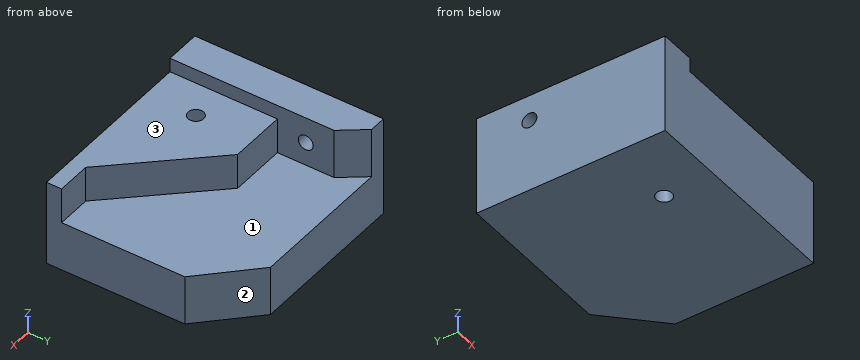
Autodesk Fusion 360 part; units mm, degrees
sketch "Sketch1" plane through (0, 0, 0) normal (0, 0, 1) x (1, 0, 0)
  line L0 (0, 0) -> (174.2555, 0)
  line L1 (174.2555, 0) -> (174.2555, 132.964)
  line L2 (174.2555, 132.964) -> (0, 132.964)
  line L3 (0, 132.964) -> (0, 0)
  line L4 (138.7597, 132.964) -> (174.2555, 97.4682)
  line L5 (138.7597, 132.964) -> (188.9583, 132.964) construction
  dimension "d1" = 45
extrude "Extrude1" add sketch "Sketch1" along normal blind 35 contours L0 L1 L2 L3 L4
extrude "Extrude2" cut 1 faces at (0, 88.6427, 11.6667) along direction (1, 0, 0) blind 25
sketch "Sketch2" plane through (0, 0, 35) normal (0, 0, 1) x (-1, 0, 0)
  line L0 (-25, -132.964) -> (-25, 0)
  line L1 (-25, 0) -> (-174.2555, 0)
  line L2 (-174.2555, 0) -> (-174.2555, -97.4682)
  line L3 (-174.2555, -97.4682) -> (-138.7597, -132.964)
  line L4 (-138.7597, -132.964) -> (-25, -132.964)
  line L5 (-25, -132.964) -> (-25, 0)
  line L6 (-50, 0) -> (-50, -110)
  line L7 (-50, -110) -> (-50, -115.7208)
  line L8 (-50, -115.7208) -> (-36.875, -132.964)
extrude "Extrude3" add sketch "Sketch2" along normal blind 35 contours L0 L1 L4 L5 L6 L7 L8
sketch "Sketch3" plane through (0, 0, 35) normal (0, 0, 1) x (-1, 0, 0)
  line L0 (-36.875, -132.964) -> (-50, -115.7208)
  line L1 (-50, -115.7208) -> (-50, 0)
  line L2 (-50, 0) -> (-174.2555, 0)
  line L3 (-174.2555, 0) -> (-174.2555, -97.4682)
  line L4 (-174.2555, -97.4682) -> (-138.7597, -132.964)
  line L5 (-138.7597, -132.964) -> (-36.875, -132.964)
  line L6 (-174.2555, -10.6135) -> (-155, -10.6135)
  line L7 (-50, 0) -> (-174.2555, 0)
  line L8 (-155, -10.6135) -> (-150, -10.6135)
  line L9 (-50, -75.7001) -> (-90, -75.7001)
  line L10 (-90, -75.7001) -> (-150, -10.6135)
extrude "Extrude4" add sketch "Sketch3" along normal blind 25 contours L1 L2 L3 L6 L7 L8 L9 L10
sketch "Sketch4" plane through (50, 0, 0) normal (1, 0, 0) x (0, 1, 0)
  line L0 (75.7001, 60) -> (75.7001, 35)
  line L1 (75.7001, 35) -> (115.7208, 35)
  line L2 (115.7208, 35) -> (115.7208, 70)
  line L3 (115.7208, 70) -> (0, 70)
  line L4 (0, 70) -> (0, 60)
  line L5 (0, 60) -> (75.7001, 60)
  circle A0 centre (95.7105, 51.6698) radius 5.2582
extrude "Extrude5" cut sketch "Sketch4" against normal blind 50 contours A0
sketch "Sketch5" plane through (0, 0, 60) normal (0, 0, 1) x (-1, 0, 0)
  line L0 (-174.2555, -10.6135) -> (-150, -10.6135)
  line L1 (-150, -10.6135) -> (-90, -75.7001)
  line L2 (-90, -75.7001) -> (-50, -75.7001)
  line L3 (-50, -75.7001) -> (-50, 0)
  line L4 (-50, 0) -> (-174.2555, 0)
  line L5 (-174.2555, 0) -> (-174.2555, -10.6135)
  circle A0 centre (-74.3342, -35.2984) radius 5.4818
extrude "Extrude6" cut sketch "Sketch5" against normal blind 150 contours A0
Verification items for the finished model (mm, model axes). Face numbers are marked on the shaded views. A direction names the side the tool comes from. Give positions to 0.01 mm unless a question says otherwise; leave off trailing zeros. Loops run counter-clockwise (first coordinate to the right, second up) from the corner with the lowest first, then second, coordinate; pieces in that order, holes last.
1. Section check A-A, the plane z = 53.5. Enter the section's corners in (x, y) (1 decimal).
2. Set-up check for the marked faces 1, 2 and 3: record each of +Z, -Z, +X, -X, +Y, -Y from which the full face is reachable in a straight line by a thin tool's end or side.
3. Section check C-C, the plane x = 72. Enter the section's corners in (y, z).
4. Section check D-D, the plane z = 38.5. Enter the section's corners in (x, y) (1 decimal), then the cut area to 3 significant figures.
5. Section check B-B, the plane y = 93.5. Enter the section's corners in (x, z).
6. Thickness scan on line 1 (Z direction, x = 123, y = 91); line 2 (Z direction, x = 99.5, y = 33); line 3 (X direction, y = 98.5, z = 64.5). Record the ranges inside material, lowest first.
7. Go/stop test with flat-tipped pins: pin 1 Ø10.5 at (y, z) = (65.5, 50) entering from +X; pin 2 Ø22.5 at (x, y) = (119.5, 43) entering from +Z; pin 3 Ø19.5 at (x, z) = (165, 45.5) entering from +Y; pin 4 Ø8 at (x, z) = (68, 19) entering from -Y. Record where each tip stops, or that it passes through.
Geometry says:
1. outline: (25, 0) - (174.3, 0) - (174.3, 10.6) - (150, 10.6) - (90, 75.7) - (50, 75.7) - (50, 90.8) - (25, 90.8) - close; (25, 100.6) - (50, 100.6) - (50, 115.7) - (36.9, 133) - (25, 133) - close; hole circle Ø11 at (74.3, 35.3)
2. face 1: +Z, +X, +Y
2. face 2: +Z, -Z, +X, +Y
2. face 3: +Z, +X, +Y, -Y
3. outline: (0, 0) - (30.34, 0) - (30.34, 60) - (0, 60) - close; (40.26, 0) - (132.96, 0) - (132.96, 35) - (75.7, 35) - (75.7, 60) - (40.26, 60) - close
4. outline: (25, 0) - (174.3, 0) - (174.3, 10.6) - (150, 10.6) - (90, 75.7) - (50, 75.7) - (50, 115.7) - (36.9, 133) - (25, 133) - close; hole circle Ø11 at (74.3, 35.3)
4. area: 8,990 mm2
5. outline: (25, 0) - (174.26, 0) - (174.26, 35) - (50, 35) - (50, 46.9) - (25, 46.9) - close; (25, 56.44) - (50, 56.44) - (50, 70) - (25, 70) - close
6. line 1: z = 0 to 35
6. line 2: z = 0 to 60
6. line 3: x = 25 to 50
7. pin 1: stops at x = 104.24
7. pin 2: stops at z = 60
7. pin 3: stops at y = 10.61
7. pin 4: stops at y = 0
